Read the model definition and answer for the solid it produces. Units are mm, in the model's axes. Give positions to 0.01 mm unless a question says otherwise; leave off trailing zeros. Write each question's results on one line, items separated by ' | '. Start each with the question number.
Q1. Given pin 1 (3 mm diameter, centred on y = -259.525, z = 36.5, fed in from -X), flat-ended and moving along its own axis, determine where the tip first touches the part or whether it passes through.
Q2. The part is cut by section A-A, the plane x = 4.25. State how many separate pieces and enclosed holes the cut face has, plus the area to 3 significant figures.
Q3. Find the intervals of material crossed by line 1 (Z direction, x = 2.25, y = -320.5); line 2 (Z direction, x = 0.75, y = -3); line 3 (Y direction, x = 0.5, z = 36.5) (3 decimals), in increasing order. Write a range as from..to.
```python
from build123d import *

# Parameters (mm, degrees)
SKETCH1_R                            = 3.3
SKETCH1_R_2                          = 1.7
SKETCH1_R_3                          = 26
BOSS_EXTRUDE1_DEPTH                  = 6.35
CUT_EXTRUDE1_DEPTH                   = 549.511460682
FILLET1_R                            = 3
SKETCH4_R                            = 1.75
CUT_EXTRUDE2_DEPTH                   = 549.511460792
SKETCH5_R                            = 1.2
CUT_EXTRUDE4_DEPTH                   = 549.511460792
BOSS_EXTRUDE2_START                  = -6.35
BOSS_EXTRUDE2_DEPTH                  = 6.35
TAP_DRILL_FOR_M3X0_5_TAP1_AT_2_COUNT = 2
TAP_DRILL_FOR_M3X0_5_TAP1_AT_2_PITCH = 13.03070812
CIRPATTERN1_COUNT                    = 2
CIRPATTERN1_ANGLE                    = 90
CUT_EXTRUDE5_DEPTH                   = 549.511460792
SKETCH10_R                           = 30
CUT_EXTRUDE6_DEPTH                   = 549.511460792


with BuildPart() as part:
    # Sketch1 → Boss-Extrude1 (new body)
    with BuildSketch(Plane(origin=(0, 0, 0), x_dir=(0, -1, 0), z_dir=(1, 0, 0))):
        with BuildLine():
            Line((0, 46.5), (500, 46.5))
            ThreePointArc((500, 46.5), (546.5, 0), (500, -46.5))
            Line((500, -46.5), (0, -46.5))
            ThreePointArc((0, -46.5), (-46.5, 0), (0, 46.5))
        make_face()
        with Locations(Location((-16, 0, 0), (0, 0, 90))):
            Circle(SKETCH1_R, mode=Mode.SUBTRACT)
        with Locations(Location((-11.313708499, 11.313708499, 0), (0, 0, 90))):
            Circle(SKETCH1_R, mode=Mode.SUBTRACT)
        with Locations(Location((0, 16, 0), (0, 0, 90))):
            Circle(SKETCH1_R, mode=Mode.SUBTRACT)
        with Locations(Location((11.313708499, 11.313708499, 0), (0, 0, 90))):
            Circle(SKETCH1_R, mode=Mode.SUBTRACT)
        with Locations(Location((16, 0, 0), (0, 0, 90))):
            Circle(SKETCH1_R, mode=Mode.SUBTRACT)
        with Locations(Location((11.313708499, -11.313708499, 0), (0, 0, 90))):
            Circle(SKETCH1_R, mode=Mode.SUBTRACT)
        with Locations(Location((537.25, 0, 0), (0, 0, 90))):
            Circle(SKETCH1_R_2, mode=Mode.SUBTRACT)
        with Locations(Location((530.13588304, -21.895000648, 0), (0, 0, 90))):
            Circle(SKETCH1_R_2, mode=Mode.SUBTRACT)
        with Locations(Location((511.51088304, -35.426855232, 0), (0, 0, 90))):
            Circle(SKETCH1_R_2, mode=Mode.SUBTRACT)
        with Locations(Location((488.48911696, -35.426855232, 0), (0, 0, 90))):
            Circle(SKETCH1_R_2, mode=Mode.SUBTRACT)
        with Locations(Location((469.86411696, -21.895000648, 0), (0, 0, 90))):
            Circle(SKETCH1_R_2, mode=Mode.SUBTRACT)
        with Locations(Location((462.75, 0, 0), (0, 0, 90))):
            Circle(SKETCH1_R_2, mode=Mode.SUBTRACT)
        with Locations(Location((469.86411696, 21.895000648, 0), (0, 0, 90))):
            Circle(SKETCH1_R_2, mode=Mode.SUBTRACT)
        with Locations(Location((488.48911696, 35.426855232, 0), (0, 0, 90))):
            Circle(SKETCH1_R_2, mode=Mode.SUBTRACT)
        with Locations(Location((511.51088304, 35.426855232, 0), (0, 0, 90))):
            Circle(SKETCH1_R_2, mode=Mode.SUBTRACT)
        with Locations(Location((530.13588304, 21.895000648, 0), (0, 0, 90))):
            Circle(SKETCH1_R_2, mode=Mode.SUBTRACT)
        with Locations(Location((500, 0, 0), (0, 0, 90))):
            Circle(SKETCH1_R_3, mode=Mode.SUBTRACT)
        with Locations(Location((0, -16, 0), (0, 0, 90))):
            Circle(SKETCH1_R, mode=Mode.SUBTRACT)
        with Locations(Location((-11.313708499, -11.313708499, 0), (0, 0, 90))):
            Circle(SKETCH1_R, mode=Mode.SUBTRACT)
    extrude(amount=BOSS_EXTRUDE1_DEPTH)

    # Sketch3 → Cut-Extrude1 (cut, through all)
    with BuildSketch(Plane(origin=(6.35, 0, 0), x_dir=(0, 0, -1), z_dir=(1, 0, 0))):
        Polygon((0, -422.848022722), (27.858212922, -368.632839363), (0, -339.139268075), (-27.858212922, -368.632839363), align=None)
        Polygon((0, -41.368651369), (-27.312924288, -58.435222232), (0, -141.248998295), (27.312924288, -58.435222232), align=None)
        Polygon((3, -313.189087212), (27.858212922, -339.506549748), (27.858212922, -258.646044282), align=None)
        Polygon((-27.858212922, -339.506549748), (-27.858212922, -258.646044282), (-3, -313.189087212), align=None)
        Polygon((-27.858212922, -401.452857349), (-11, -434.260816252), (-27.858212922, -461.481824785), align=None)
        Polygon((11, -434.260816252), (27.858212922, -461.481824785), (27.858212922, -401.452857349), align=None)
        with BuildLine():
            Line((0, -164.248853344), (-27.858212922, -178.200474573))
            add(Edge.make_bspline(
                [(-27.858212922, -178.200474573), (-43.7790539, -216.093343216), (-18.61661693, -258.276071598), (0, -289.085024731)],
                knots=[0, 0, 0, 0, 1, 1, 1, 1], degree=3))
            add(Edge.make_bspline(
                [(27.858212922, -178.200474573), (43.7790539, -216.093343216), (18.61661693, -258.276071598), (0, -289.085024731)],
                knots=[0, 0, 0, 0, 1, 1, 1, 1], degree=3))
            Line((27.858212922, -178.200474573), (0, -164.248853344))
        make_face()
        Polygon((7.5, -156.820958214), (27.312924288, -96.747453897), (27.312924288, -166.743432993), align=None)
        Polygon((-27.312924288, -96.747453897), (-27.312924288, -166.743432993), (-7.5, -156.820958214), align=None)
    extrude(amount=-CUT_EXTRUDE1_DEPTH, mode=Mode.SUBTRACT)

    # Fillet1
    fillet1_edges = [part.edges().sort_by_distance(p)[0] for p in [
        (3.175, -58.435222232, -27.312924288),
        (3.175, -41.368651369, 0),
        (3.175, -58.435222232, 27.312924288),
        (3.175, -141.248998295, 0),
        (3.175, -289.085024731, 0),
        (3.175, -164.248853344, 0),
        (3.175, -401.452857349, 27.858212922),
        (3.175, -434.260816252, 11),
        (3.175, -461.481824785, 27.858212922),
        (3.175, -461.481824785, -27.858212922),
        (3.175, -434.260816252, -11),
        (3.175, -401.452857349, -27.858212922),
        (3.175, -368.632839363, -27.858212922),
        (3.175, -339.139268075, 0),
        (3.175, -368.632839363, 27.858212922),
        (3.175, -422.848022722, 0),
        (3.175, -313.189087212, 3),
        (3.175, -339.506549748, 27.858212922),
        (3.175, -258.646044282, 27.858212922),
        (3.175, -178.200474573, -27.858212922),
        (3.175, -178.200474573, 27.858212922),
        (3.175, -339.506549748, -27.858212922),
        (3.175, -313.189087212, -3),
        (3.175, -258.646044282, -27.858212922),
        (3.175, -96.747453897, 27.312924288),
        (3.175, -166.743432993, 27.312924288),
        (3.175, -156.820958214, 7.5),
        (3.175, -166.743432993, -27.312924288),
        (3.175, -156.820958214, -7.5),
        (3.175, -96.747453897, -27.312924288),
    ]]
    fillet(fillet1_edges, radius=FILLET1_R)

    # Sketch4 → Cut-Extrude2 (cut, through all)
    with BuildSketch(Plane(origin=(6.35, 0, 0), x_dir=(0, 0, -1), z_dir=(1, 0, 0))):
        with Locations((-36.5, -103.175)):
            Circle(SKETCH4_R)
        with Locations(Location((36.5, -103.175, 0), (0, 0, 180))):
            Circle(SKETCH4_R)
        with Locations(Location((-36.5, -259.525, 0), (0, 0, 180))):
            Circle(SKETCH4_R)
        with Locations((36.5, -259.525)):
            Circle(SKETCH4_R)
        with Locations((-36.5, -415.875)):
            Circle(SKETCH4_R)
        with Locations(Location((36.5, -415.875, 0), (0, 0, 180))):
            Circle(SKETCH4_R)
    extrude(amount=-CUT_EXTRUDE2_DEPTH, mode=Mode.SUBTRACT)

    # Sketch5 → Cut-Extrude4 (cut, through all)
    with BuildSketch(Plane(origin=(6.35, 0, 0), x_dir=(0, 0, -1), z_dir=(1, 0, 0))):
        with Locations((-6.916110339, -463.343078174)):
            Circle(SKETCH5_R)
        with Locations((-15.951147244, -466.27873962)):
            Circle(SKETCH5_R)
    extrude(amount=-CUT_EXTRUDE4_DEPTH, mode=Mode.SUBTRACT)

    # Sketch6 → Boss-Extrude2 (add)
    with BuildSketch(Plane(origin=(6.35, 0, 0), x_dir=(0, 0, -1), z_dir=(1, 0, 0)).offset(BOSS_EXTRUDE2_START)):
        with BuildLine():
            Line((-44.110383395, -529.968247771), (-29.968247771, -544.110383395))
            ThreePointArc((-29.968247771, -544.110383395), (-23.286397782, -542.399293624), (-16.474718596, -543.483717035))
            ThreePointArc((-16.474718596, -543.483717035), (-32.880465325, -532.880465325), (-43.483717035, -516.474718596))
            ThreePointArc((-43.483717035, -516.474718596), (-42.399293624, -523.286397782), (-44.110383395, -529.968247771))
        make_face()
    boss_extrude2 = extrude(amount=BOSS_EXTRUDE2_DEPTH)

    # Sketch8 → Tap Drill for M3x0.5 Tap1 (revolve, cut)
    with BuildSketch(Plane(origin=(3.175, -532.796674896, 41.28195627), x_dir=(0, -0.7071067811865424, -0.7071067811865527), z_dir=(1, 0, 0))):
        Polygon((0, 0), (0, 5.751075774), (1.25, 5), (1.25, 0), align=None)
    tap_drill_for_m3x0_5_tap1 = revolve(axis=Axis((3.175, -537.286802956, 45.772084331), (0, 0.7071067811865529, -0.7071067811865422)), mode=Mode.SUBTRACT)

    # Tap Drill for M3x0.5 Tap1 at 2: Tap Drill for M3x0.5 Tap1 ×2
    with Locations(*[Vector(0, -0.7071067811865422, -0.7071067811865529) * (i * TAP_DRILL_FOR_M3X0_5_TAP1_AT_2_PITCH) for i in range(1, TAP_DRILL_FOR_M3X0_5_TAP1_AT_2_COUNT)]):
        add(tap_drill_for_m3x0_5_tap1, mode=Mode.SUBTRACT)

    # CirPattern1: Boss-Extrude2, Tap Drill for M3x0.5 Tap1 ×2 about axis
    cirpattern1_axis = Axis((0, -500, 0), (1, 0, 0))
    add([boss_extrude2.rotate(cirpattern1_axis, i * CIRPATTERN1_ANGLE / (CIRPATTERN1_COUNT - 1)) for i in range(1, CIRPATTERN1_COUNT)])
    add([tap_drill_for_m3x0_5_tap1.rotate(cirpattern1_axis, i * CIRPATTERN1_ANGLE / (CIRPATTERN1_COUNT - 1)) for i in range(1, CIRPATTERN1_COUNT)], mode=Mode.SUBTRACT)

    # CirPattern1 copy 1 sketch → CirPattern1 copy 1 (revolve, cut)
    with BuildSketch(Plane(origin=(3.175, -532.067854195, -42.010776971), x_dir=(0, 0.7071067811865551, -0.7071067811865399), z_dir=(1, 0, 0))):
        Polygon((0, 0), (0, 5.751075774), (1.25, 5), (1.25, 0), align=None)
    revolve(axis=Axis((3.175, -536.557982255, -46.500905032), (0, 0.7071067811865398, 0.7071067811865553)), mode=Mode.SUBTRACT)

    # Sketch9 → Cut-Extrude5 (cut, through all)
    with BuildSketch(Plane(origin=(6.35, 0, 0), x_dir=(0, 0, -1), z_dir=(1, 0, 0))):
        with BuildLine():
            Line((-43.483717035, -516.474718596), (-63.483717035, -516.474718596))
            ThreePointArc((-63.483717035, -516.474718596), (0, -565.586573942), (63.483717035, -516.474718596))
            Line((63.483717035, -516.474718596), (43.483717035, -516.474718596))
            ThreePointArc((43.483717035, -516.474718596), (0, -546.5), (-43.483717035, -516.474718596))
        make_face()
    extrude(amount=-CUT_EXTRUDE5_DEPTH, mode=Mode.SUBTRACT)

    # Sketch10 → Cut-Extrude6 (cut, through all)
    with BuildSketch(Plane(origin=(6.35, 0, 0), x_dir=(0, 0, -1), z_dir=(1, 0, 0))):
        with Locations((0, -500)):
            Circle(SKETCH10_R)
    extrude(amount=-CUT_EXTRUDE6_DEPTH, mode=Mode.SUBTRACT)


solid = part.part
```
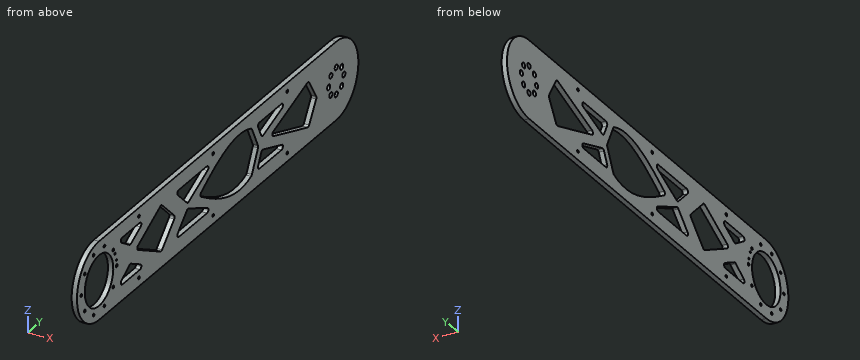
Check sheet entries:
1) pin 1: passes through
2) separate pieces: 1 | enclosed holes: 36 | area: 35,300 mm^2
3) line 1: z = -46.5..-27.86, -9.91..9.91, 27.86..46.5 | line 2: z = -46.5..-17.37, -14.63..14.63, 17.37..46.5 | line 3: y = -528.81..-512.829, -510.192..-489.808, -487.171..-417.625, -414.125..-261.275, -257.775..-104.925, -101.425..28.81
